Geometry check sheet. Reference: the model listing, model coordinates, mm. A direction names the side the tool comes from. Give positions to 0.01 mm unless a question says otherwise; leave off trailing zeros. Loops run counter-clockwise (first coordinate to the right, second up) from the corner with the lowest first, then second, coordinate; pieces in that order, holes last. Notation, with made-up numbers: (21.5, 31.5) -> (79.5, 31.5) arc R33 cw to (79.5, 67.5) -> close; hole circle Ø9 at (47.25, 81.5). An arc over 180 degrees is marked (long way). Write item = value, one per line.
Autodesk Inventor part; units mm, degrees
ref_plane "YZ Plane" through (0, 0, 0) normal (1, 0, 0) x (0, 1, 0)
ref_plane "XZ Plane" through (0, 0, 0) normal (0, 1, 0) x (-1, 0, 0)
ref_plane "XY Plane" through (0, 0, 0) normal (0, 0, 1) x (1, 0, 0)
sketch "スケッチ1" plane through (0, 0, 0) normal (0, 0, 1) x (1, 0, 0)
  line L0 (0, -5.5) -> (0.95, -5.5)
  line L1 (0.95, -5.5) -> (1.25, -5.2)
  line L2 (1.25, -5.2) -> (1.25, 0)
  line L3 (1.25, 0) -> (1.25, 0)
  line L4 (1.25, 0) -> (1.25, 0.5)
  line L5 (1.25, 0.5) -> (2.7, 0.5)
  line L6 (3, 11.2) -> (2.7, 11.5)
  line L7 (2.7, 11.5) -> (1.55, 11.5)
  line L8 (1.55, 11.5) -> (1.25, 11.2)
  line L9 (0, 7.4044) -> (0, -7.4044) construction
  line L10 (0, -5.5) -> (0, 5.5)
  line L11 (0, 5.5) -> (1.25, 5.5)
  line L12 (1.25, 5.5) -> (1.25, 11.2)
  line L13 (2.7, 0.5) -> (3, 0.8)
  line L14 (3, 0.8) -> (3, 11.2)
  point P0 (0, 0)
  point P1 (0, 0)
  dimension "d0" = 2.5
  dimension "d1" = 6
  dimension "d2" = 0.3
  dimension "d3" = 0.3
  dimension "d4" = 2.5
  dimension "d5" = 0.5
  dimension "d6" = 11
  dimension "d8" = 0.3
  dimension "d9" = 2.5
  dimension "d10" = 6
  dimension "d11" = 0.3
  dimension "d12" = 0.3
  dimension "d13" = 0.3
  dimension "d14" = 0.3
  dimension "d15" = 6
revolve "回転1" add sketch "スケッチ1" angle 360 about axis through (0, 7.4044, 0) along (0, -1, 0)
sketch "スケッチ2" plane through (0, -5.5, 0) normal (0, -1, 0) x (1, 0, 0)
  circle A0 centre (0, 0) radius 0.95
  circle A1 centre (0, 0) radius 9.0242
extrude "押し出し1" cut sketch "スケッチ2" against normal blind 0.5 contours A0 | A1
sketch "スケッチ3" plane through (0, 11.5, 0) normal (0, 1, 0) x (1, 0, 0)
  circle A0 centre (0, 0) radius 3
  line L0 (3, 0) -> (-3, 0)
  line L1 (-3, -0.5) -> (-3, 0.5)
  line L2 (3, -0.5) -> (-3, -0.5)
  line L3 (3, 0.5) -> (-3, 0.5)
  line L4 (3, -0.5) -> (3, 0.5)
  point P0 (0, 0)
  point P1 (-2.958, -0.5)
  point P2 (2.958, -0.5)
  point P3 (2.958, 0.5)
  point P4 (-2.958, 0.5)
  dimension "d22" = 0.5
  dimension "d23" = 0.5
extrude "押し出し2" cut sketch "スケッチ3" against normal blind 1 contours L0 A0 L3 | A0 L2 L0
equation "\"d3\" = d2"
equation "\"d11\" = d8"
equation "\"d12\" = d8"
equation "\"d13\" = d12"
equation "\"d14\" = d13"
properties part number "BRU-312S" material "ステンレス鋼 AISI 304"
Item 1: Draft check along X on faces 1 (the flat face through (0, 5.5, 0)), 2 (the flat face through (0, 11.5, -2)), 3 (the cylindrical face through (2.86, 6.07, -0.9)). Enter one of: +X half, -X half, draft (parallel to the pull), parting line (faces both ways), or undercut.
Answer:
face_1 = undercut
face_2 = draft
face_3 = parting line
Item 2: Section check D-D, the plane y = 4.75. Record the cut outline in (x, z).
Answer:
outline = circle Ø6 at (0, 0)
Item 3: Thickness scan on L1, parallel to Z at x = 0, y = 8.5; L2, parallel to X at y = -4.5, z = 0.1; L3, parallel to Y at x = -1, z = -1.2. Record the ranges inside material, lowest first. Write a range as [from, to].
Answer:
L1 = [-3, -1.25], [1.25, 3]
L2 = [-1.25, 1.25]
L3 = [0.5, 11.5]
Item 4: Tool access check on faces 4 (the conical face through (-0.02, 11.32, 1.37)), 5 (the flat face through (0, -5, 0)), 6 (the flat face through (2, 11, -0.5)), 7 (the cylindrical face through (-0.27, -2.21, 1.22)). Record the directions out of +Z, -Z, +X, -X, +Y, -Y that give a thin tool (end or side, any length) a straight path to the whole face; none if there is none.
Answer:
face_4 = +Y
face_5 = +Z, -Z, +X, -X, -Y
face_6 = +X, -X, +Y
face_7 = -Y
Item 5: Section check B-B, the plane x = 0. Record the cut outline in (y, z), plus the area to 3 significant figures.
Answer:
outline = (-5, -1.25) -> (0.5, -1.25) -> (0.5, -2.7) -> (0.8, -3) -> (11.2, -3) -> (11.5, -2.7) -> (11.5, -1.55) -> (11.2, -1.25) -> (5.5, -1.25) -> (5.5, 1.25) -> (11.2, 1.25) -> (11.5, 1.55) -> (11.5, 2.7) -> (11.2, 3) -> (0.8, 3) -> (0.5, 2.7) -> (0.5, 1.25) -> (-5, 1.25) -> close
area = 64.5 mm^2
Item 6: Section check A-A, the plane z = 0. Record the cut outline in (x, y), plus the area to 3 significant figures.
Answer:
outline = (-3, 0.8) -> (-2.7, 0.5) -> (-1.25, 0.5) -> (-1.25, -5) -> (1.25, -5) -> (1.25, 0.5) -> (2.7, 0.5) -> (3, 0.8) -> (3, 10.5) -> (1.25, 10.5) -> (1.25, 5.5) -> (-1.25, 5.5) -> (-1.25, 10.5) -> (-3, 10.5) -> close
area = 61.2 mm^2
Item 7: Gauge pin test, flat ends, axial feed: pin 1 (2 mm diameter, centred on x = 1.5, z = -2, fed in from -Y); pin 2 (3 mm diameter, centred on x = 0, z = 0, fed in from +Y); pin 3 (0.5 mm diameter, centred on x = 2, y = 11, fed in from +Z). Record the tip position at first contact, or that the pin passes through.
Answer:
pin_1 = 0.5
pin_2 = 11.45
pin_3 = 2.44
Item 8: Section check C-C, the plane y = 7. Record the cut outline in (x, z), plus the area to 3 significant figures.
Answer:
outline = circle Ø6 at (0, 0); hole circle Ø2.5 at (0, 0)
area = 23.4 mm^2
